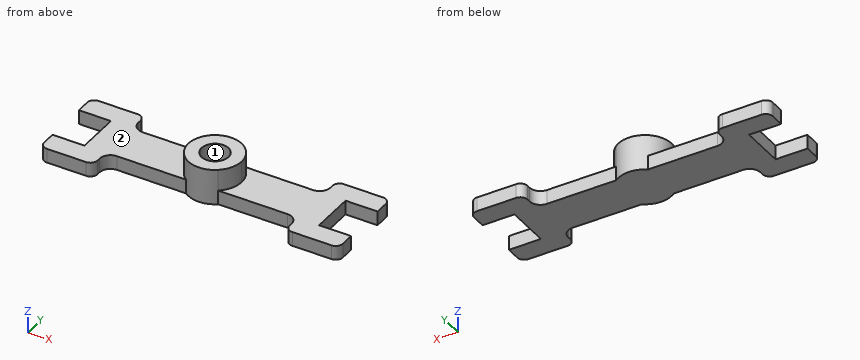
```python
from build123d import *

# Parameters (mm, degrees)
F0_R     = 3.8
F1_DEPTH = 10
F2_DEPTH = 4
F3_DEPTH = 3


with BuildPart() as f1:
    # F0 (on Top) → F1 (new body)
    with BuildSketch(Plane.XY):
        with BuildLine():
            ThreePointArc((7.5, 0), (6.7082039325, 3.3541019662), (4.5, 6))
            Line((4.5, 6), (-4.5, 6))
            ThreePointArc((-4.5, 6), (-7.5, 0), (-4.5, -6))
            Line((-4.5, -6), (4.5, -6))
            ThreePointArc((4.5, -6), (6.7082039325, -3.3541019662), (7.5, 0))
        make_face()
        Circle(F0_R, mode=Mode.SUBTRACT)
        with BuildLine():
            Line((4.5, -6), (-4.5, -6))
            ThreePointArc((-4.5, -6), (0, -7.5), (4.5, -6))
        make_face()
        with BuildLine():
            Line((-4.5, 6), (4.5, 6))
            ThreePointArc((4.5, 6), (0, 7.5), (-4.5, 6))
        make_face()
    extrude(amount=F1_DEPTH)

    # F0 (on Top) → F2 (join)
    with BuildSketch(Plane.XY):
        with BuildLine():
            ThreePointArc((-4.5, -6), (-7.5, 0), (-4.5, 6))
            Line((-4.5, 6), (-24, 6))
            ThreePointArc((-24, 6), (-26.1213203436, 6.8786796564), (-27, 9))
            Line((-27, 9), (-27, 10))
            ThreePointArc((-27, 10), (-27.5857864376, 11.4142135624), (-29, 12))
            Line((-29, 12), (-40, 12))
            ThreePointArc((-40, 12), (-41.4142135624, 11.4142135624), (-42, 10))
            Line((-42, 10), (-42, 6.15))
            Line((-42, 6.15), (-33, 6.15))
            Line((-33, 6.15), (-33, -6.15))
            Line((-33, -6.15), (-42, -6.15))
            Line((-42, -6.15), (-42, -10))
            ThreePointArc((-42, -10), (-41.4142135624, -11.4142135624), (-40, -12))
            Line((-40, -12), (-29, -12))
            ThreePointArc((-29, -12), (-27.5857864376, -11.4142135624), (-27, -10))
            Line((-27, -10), (-27, -9))
            ThreePointArc((-27, -9), (-26.1213203436, -6.8786796564), (-24, -6))
            Line((-24, -6), (-4.5, -6))
        make_face()
        with BuildLine():
            ThreePointArc((27, 9), (26.1213203436, 6.8786796564), (24, 6))
            Line((24, 6), (4.5, 6))
            ThreePointArc((4.5, 6), (6.7082039325, 3.3541019662), (7.5, 0))
            ThreePointArc((7.5, 0), (6.7082039325, -3.3541019662), (4.5, -6))
            Line((4.5, -6), (24, -6))
            ThreePointArc((24, -6), (26.1213203436, -6.8786796564), (27, -9))
            Line((27, -9), (27, -10))
            ThreePointArc((27, -10), (27.5857864376, -11.4142135624), (29, -12))
            Line((29, -12), (40, -12))
            ThreePointArc((40, -12), (41.4142135624, -11.4142135624), (42, -10))
            Line((42, -10), (42, -6.15))
            Line((42, -6.15), (33, -6.15))
            Line((33, -6.15), (33, 6.15))
            Line((33, 6.15), (42, 6.15))
            Line((42, 6.15), (42, 10))
            ThreePointArc((42, 10), (41.4142135624, 11.4142135624), (40, 12))
            Line((40, 12), (29, 12))
            ThreePointArc((29, 12), (27.5857864376, 11.4142135624), (27, 10))
            Line((27, 10), (27, 9))
        make_face()
    extrude(amount=F2_DEPTH)

    # F0 (on Top) → F3 (join)
    with BuildSketch(Plane.XY):
        Circle(F0_R)
    extrude(amount=F3_DEPTH)


solid = f1.part
```
Can you work these out from the model? Positions are in its coordinate system, mm. Face numbers are marked on the shaded views. Give positions to 0.01 mm unless a question says otherwise; leave off trailing zeros. Write each loop counter-clockwise with the first axis right and the second up, starting at its lowest first coordinate (ties: lowest second). Pieces come first, ordered by that corner, then holes. Notation, with made-up numbers: (30, 42.25) -> (65, 42.25) arc R10 cw to (65, 58.25) -> close; hole circle Ø3 at (79.5, 57). An arc over 180 degrees is marked (long way). One line per item, written item: value.
Q1. Imagine slicing it at C-C on x = 17. Please give me the cut outline in (y, z).
Results found:
outline: (-6, 0) -> (6, 0) -> (6, 4) -> (-6, 4) -> close
Q2. Imagine slicing it at D-D on y = -5.25. Please give me the cut outline in (x, z), and give its area (3 significant figures).
Results found:
outline: (-33, 0) -> (33, 0) -> (33, 4) -> (5.36, 4) -> (5.36, 10) -> (-5.36, 10) -> (-5.36, 4) -> (-33, 4) -> close
area: 328 mm^2
Q3. Imagine slicing it at A-A on x = 0. Please give me the cut outline in (y, z).
Results found:
outline: (-7.5, 0) -> (7.5, 0) -> (7.5, 10) -> (3.8, 10) -> (3.8, 3) -> (-3.8, 3) -> (-3.8, 10) -> (-7.5, 10) -> close
Q4. Please list where these lines run through material, in increasing order: line 1 (Y direction, x = 0, z = 6); line 2 (Z direction, x = -15.5, y = -1.75); line 3 (X direction, y = -3.5, z = 9.25). Write a range as [from, to].
Results found:
line 1: y = [-7.5, -3.8], [3.8, 7.5]
line 2: z = [0, 4]
line 3: x = [-6.63, -1.48], [1.48, 6.63]
Q5. Imagine slicing it at B-B on y = 2.25. Please give me the cut outline in (x, z), and give its area (3 significant figures).
Results found:
outline: (-33, 0) -> (33, 0) -> (33, 4) -> (7.15, 4) -> (7.15, 10) -> (3.06, 10) -> (3.06, 3) -> (-3.06, 3) -> (-3.06, 10) -> (-7.15, 10) -> (-7.15, 4) -> (-33, 4) -> close
area: 307 mm^2
Q6. We'd pull the mould along Y, two halves only. Please class the marked faces 1 and 2: +Y half, -Y half, draft (parallel to the pull), parting line (faces both ways), or undercut.
Results found:
face 1: undercut
face 2: draft
Q7. For P1, Ø5, axis at x = -12.5, y = 2.5, coming from the +Z side; P2, Ø4, axis at y = 2, z = 8.5, coming from the +X side; P3, Ø3, axis at x = -10, z = 2, coming from the -Y side, each with a flat end and sliding along its axis, tell me the tip position at first contact or that it passes through.
Results found:
P1: stops at z = 4
P2: stops at x = 7.5
P3: stops at y = -6
